Check sheet for the modelled part. Datum: model origin and axes. Units: mm. A direction names the side the tool comes from. Round coordinates to 2 decimals unless told otherwise and drop trailing zeros. Order: outer loops, then holes, each group sorted by start corner. A loop starts at its lowest first (then second) coordinate and runs counter-clockwise, first axis right, second up.
Q1. Cross-section at A-A on z = -19.8. Record the cut outline in (x, y), then the cut area to 3 significant figures.
Q2. Cross-section at C-C on x = -16. Record the cut outline in (y, z), then the cut area to 3 significant figures.
Q3. Cross-section at B-B on y = 1.35. Record the cut outline in (x, z), then the cut area to 3 significant figures.
Q4. Scan lines: probe 1 along X at (y, z) = (3.9, -19.8); probe 2 along X at (y, z) = (3.8, -21.5); probe 3 along Z at (x, y) = (-10.5, 4.65). Record each from-to range of solid material in increasing order.
Q5. Set-up check for faces 1 (the flat face through (3, 3, -7)), 2 (the flat face through (7, 3, -34)), 3 (the flat face through (10, 3, -2.5)), 4 (the flat face through (7, 3, -5)), 5 (the flat face through (-5, 3, 6)): record each of +Z, -Z, +X, -X, +Y, -Y from which the full face is reachable in a straight line by a thin tool's end or side.
Q6. Depth check by flat-ended pin: P1, Ø2, axis at x = -28.5, z = -0.5, coming from the -Y side; P2, Ø1.1, axis at y = 4.5, z = 4.5, coming from the -X side; P3, Ø3, axis at y = 2, z = 3, coming from the +X side; P4, Ø1.8, axis at x = 10, y = 4, coming from the -Z side. Enter the tip coordinate at first touch or a pass-through.
Q7. Mould release check, pull along X, two halves, no side actions. Record for faces 6 (the flat face through (0, 3, -3)), 7 (the flat face through (2, 3, 0)), 8 (the flat face through (-14, 3, 4)): +X half, -X half, draft (parallel to the pull), parting line (faces both ways), or undercut.
from build123d import *

# Parameters (mm, degrees)
SKETCH1_R           = 11
BOSS_EXTRUDE1_DEPTH = 6


with BuildPart() as part:
    # Sketch1 → Boss-Extrude1 (new body)
    with BuildSketch(Plane(origin=(0, 0, 0), x_dir=(1, 0, 0), z_dir=(0, 1, 0))):
        with BuildLine():
            Line((0, 0), (0, 7))
            Line((0, 7), (7, 7))
            Line((7, 7), (7, 2.5))
            Line((7, 2.5), (13, 2.5))
            Line((13, 2.5), (13, 27))
            Line((13, 27), (7, 27))
            Line((7, 27), (7, 41.8))
            Line((7, 41.8), (-14, 41.8))
            ThreePointArc((-14, 41.8), (-36, 19.8), (-14, -2.2))
            Line((-14, -2.2), (-14, -6))
            Line((-14, -6), (4.5, -6))
            Line((4.5, -6), (4.5, 0))
            Line((4.5, 0), (0, 0))
        make_face()
        with Locations(Location((-14, 19.8, 0), (0, 0, 270))):
            Circle(SKETCH1_R, mode=Mode.SUBTRACT)
    extrude(amount=BOSS_EXTRUDE1_DEPTH)


solid = part.part
Results found:
1. outline: (-36, 0) - (-25, 0) - (-25, 6) - (-36, 6) - close; (-3, 0) - (13, 0) - (13, 6) - (-3, 6) - close
1. area: 162 mm2
2. outline: (0, -41.71) - (6, -41.71) - (6, -30.62) - (0, -30.62) - close; (0, -8.98) - (6, -8.98) - (6, 2.11) - (0, 2.11) - close
2. area: 133 mm2
3. outline: (-14, -41.8) - (7, -41.8) - (7, -27) - (13, -27) - (13, -2.5) - (7, -2.5) - (7, -7) - (0, -7) - (0, 0) - (4.5, 0) - (4.5, 6) - (-14, 6) - (-14, 2.2) arc R22 ccw to start; hole circle Ø22 at (-14, -19.8)
3. area: 1,470 mm2
4. probe 1: x = -36 to -25, -3 to 13
4. probe 2: x = -35.93 to -24.87, -3.13 to 13
4. probe 3: z = -41.8 to -30.23, -9.37 to 6
5. face 1: +Y, -Y
5. face 2: -Z, +X, +Y, -Y
5. face 3: +Z, +X, +Y, -Y
5. face 4: +Z, +Y, -Y
5. face 5: +Z, +X, -X, +Y, -Y
6. P1: passes through
6. P2: stops at x = -14
6. P3: stops at x = 4.5
6. P4: stops at z = -27
7. face 6: undercut
7. face 7: draft
7. face 8: -X half
